Read the model definition and answer for the solid it produces. Units are mm, in the model's axes. Face numbers are marked on the shaded views. A direction names the side the tool comes from. Give positions to 0.01 mm unless a question says otherwise; leave off trailing zeros. Loops run counter-clockwise (first coordinate to the right, second up) from the corner with the lowest first, then second, coordinate; pieces in that order, holes last. Notation, with made-up numbers: (15.5, 45) -> (64.5, 45) arc R11 cw to (64.5, 53) -> close; hole circle Ø1 at (75, 13). An arc over 180 degrees is marked (long way). Write each question's results on one line, items separated by ' | '. Start each with the question number.
Item 1: Section A-A on x = 0 is taken. Write down the section's boundary in (y, z), and give its area (3 significant figures).
Item 2: Find the intervals of material crossed by line 1 (X direction, y = -1.5, z = -1.5); line 2 (Z direction, x = 0.75, y = 3.25); line 3 (Z direction, x = 2.5, y = -1.25), in increasing order.
Item 3: Section C-C on z = -5.5 is taken. Write down the section's boundary in (x, y), and give its area (3 significant figures).
Item 4: Which of the six approach directions +Z, -Z, +X, -X, +Y, -Y give full straight-line access (tool end or side, diameter ignored) to the marked faces 1 and 2?
Item 5: This flat-tipped pin is pushed along its axis until it touches: P1, Ø3, axis at x = -2.5, z = -4.5, coming from the -Y side. Where does it stop, or does it pass through?
Item 6: Section B-B on z = 1.5 is taken. Write down the section's boundary in (x, y).
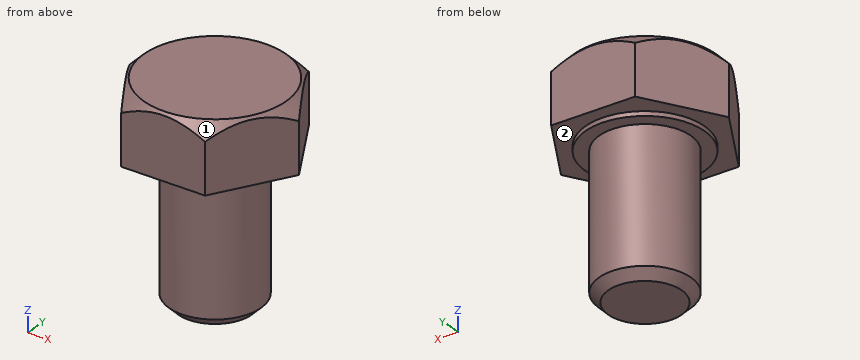
```python
from build123d import *

# Parameters (mm, degrees)
BOSS_EXTRUDE1_DEPTH = 3.5
SKETCH3_R           = 3.25
BOSS_EXTRUDE3_DEPTH = 0.25
SKETCH2_R           = 2.5
BOSS_EXTRUDE2_DEPTH = 8
CHAMFER1_SIZE       = 0.5


with BuildPart() as part:
    # Sketch1 → Boss-Extrude1 (new body)
    with BuildSketch(Plane.XY):
        Polygon((4.618802154, 0), (2.309401077, 4), (-2.309401077, 4), (-4.618802154, 0), (-2.309401077, -4), (2.309401077, -4), align=None)
    extrude(amount=BOSS_EXTRUDE1_DEPTH)

    # Sketch3 → Boss-Extrude3 (add)
    with BuildSketch(Plane(origin=(0, 0, 0), x_dir=(-1, 0, 0), z_dir=(0, 0, -1))):
        Circle(SKETCH3_R)
    extrude(amount=BOSS_EXTRUDE3_DEPTH)

    # Sketch2 → Boss-Extrude2 (add)
    with BuildSketch(Plane(origin=(0, 0, 0), x_dir=(-1, 0, 0), z_dir=(0, 0, -1))):
        Circle(SKETCH2_R)
    extrude(amount=BOSS_EXTRUDE2_DEPTH)

    # Chamfer1
    chamfer1_edges = [part.edges().sort_by_distance(p)[0] for p in [
        (2.5, 0, -8),
    ]]
    chamfer(chamfer1_edges, length=CHAMFER1_SIZE)

    # Sketch4 → Cut-Revolve1 (revolve, cut)
    with BuildSketch(Plane(origin=(0, 0, 0), x_dir=(1, 0, 0), z_dir=(0, 1, 0))):
        Polygon((-4.868802154, -3.75), (-4.868802154, -2.5), (-3.618802154, -3.75), align=None)
    revolve(axis=Axis((0, 0, 3.5), (0, 0, -1)), mode=Mode.SUBTRACT)


solid = part.part
```
Findings:
1) outline: (-4, 0) -> (-3.25, 0) -> (-3.25, -0.25) -> (-2.5, -0.25) -> (-2.5, -7.5) -> (-2, -8) -> (2, -8) -> (2.5, -7.5) -> (2.5, -0.25) -> (3.25, -0.25) -> (3.25, 0) -> (4, 0) -> (4, 3.37) -> (3.87, 3.5) -> (-3.87, 3.5) -> (-4, 3.37) -> close | area: 68.1 mm2
2) line 1: -2 to 2 | line 2: 0 to 3.5 | line 3: -0.25 to 3.5
3) outline: circle Ø5 at (0, 0) | area: 19.6 mm2
4) face 1: +Z | face 2: -Z
5) P1: y = -2.29
6) outline: (-4.62, 0) -> (-2.31, -4) -> (2.31, -4) -> (4.62, 0) -> (2.31, 4) -> (-2.31, 4) -> close
